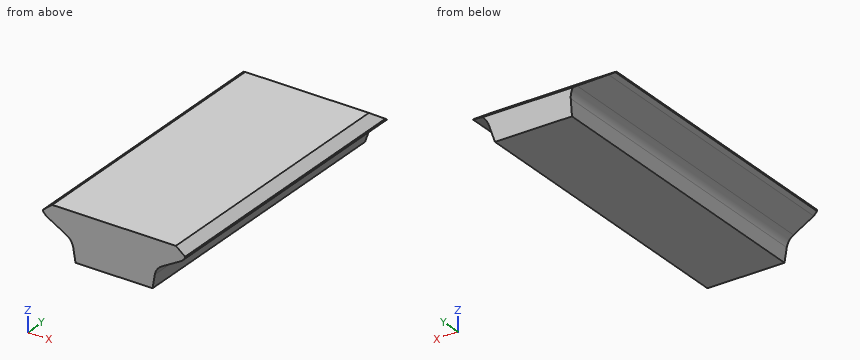
from build123d import *

# Parameters (mm, degrees)
F1_DEPTH    = 459.4
F2_SIZE2    = 31.5
F2_SIZE     = 11.8
F3_T1_DEPTH = 453.6970794399
F4_R        = 20


# Not quite as in the source:
# - a fillet or chamfer that OpenCascade refuses, or shapes differently, is made with other operations: its cross-section is extruded or revolved along the edge and cut away or added


with BuildPart() as f1:
    # F0 (on Front) → F1 (new body)
    with BuildSketch(Plane.XZ):
        Polygon((-61.18, 29.2), (-56.25, 0), (56.25, 0), (61.18, 29.2), (99, 50.6), (103.7, 55.8), (103.7, 57.8), (90.23, 68.48), (-90.23, 68.48), (-103.7, 57.8), (-103.7, 55.8), (-99, 50.6), align=None)
    extrude(amount=F1_DEPTH)

    # F2
    f2_edges = [f1.edges().sort_by_distance(p)[0] for p in [
        (0, 0, 0),
    ]]
    f2_side = f1.faces().sort_by_distance((0, -229.7, 0))[0]
    chamfer(f2_edges, length=F2_SIZE, length2=F2_SIZE2, reference=f2_side)

    # F3: chamfer of 52.9 x 37 on 1 edges, made by hand

    # F3_s2 → F3_t1 (cut)
    with BuildSketch(Plane.YZ.offset(-226.8485397199)):
        Polygon((0, 31.48), (-52.9, 68.48), (0, 68.48), align=None)
    extrude(amount=F3_T1_DEPTH, mode=Mode.SUBTRACT)

    # F4 (call 1 of 2: OpenCascade refuses the feature's edges together)
    f4_edges = [f1.edges().sort_by_distance(p)[0] for p in [
        (61.18, -230.130794, 29.2),
    ]]
    fillet(f4_edges, radius=F4_R)

    # F4#2 (call 2 of 2)
    f4_2_edges = [f1.edges().sort_by_distance(p)[0] for p in [
        (-61.18, -230.130794, 29.2),
    ]]
    fillet(f4_2_edges, radius=F4_R)


solid = f1.part
Source: CAD feature listing. Evaluate the final solid. Frame: model axes, mm. Round coordinates to 2 decimals unless told otherwise and drop trailing zeros. Loops run counter-clockwise (first coordinate to the right, second up) from the corner with the lowest first, then second, coordinate; pieces in that order, holes last. Notation, with made-up numbers: (49, 64) -> (67, 64) arc R13 ccw to (67, 85) -> close; hole circle Ø9 at (33.5, 25). An arc over 180 degrees is marked (long way). Answer as a JSON object with one key per item and string values. Group by question number.
Q1. Section query A-A (y = -374). Output: boundary loops of the cut face in (x, z), plus the area to 3 significant figures.
Q2. Ray query, line 1 (Y direction, x = 3.5, z = 36.5); line 2 (X direction, y = -176, z = 27.5); line 3 (Y direction, x = 57, z = 44.5). Return the intervals inside material, ascending. Write a range as from..to.
Q3. Section query B-B (x = 15). Output: boundary loops of the cut face in (y, z), plus the area to 3 significant figures.
Q4. Section query D-D (x = 83). Output: boundary loops of the cut face in (y, z).
Q5. Contact query for flat-ended pins moving along their axis: P1, Ø10, axis at y = -78.5, z = 34, coming from the +X side; P2, Ø3, axis at y = -361, z = 28.5, coming from the +X side; P3, Ø6, axis at y = -367.5, z = 10, coming from the -X side. Output: stop coordinate, or through.
Q6. Section query C-C (z = 8). Output: boundary loops of the cut face in (x, y).
Completed:
{
 "1": {"outline": "(-103.7, 55.8) -> (-99, 50.6) -> (-69.47, 33.89) arc R20 cw to (-59.59, 19.81) -> (-56.25, 0) -> (56.25, 0) -> (59.59, 19.81) arc R20 cw to (69.47, 33.89) -> (99, 50.6) -> (103.7, 55.8) -> (103.7, 57.8) -> (90.23, 68.48) -> (-90.23, 68.48) -> (-103.7, 57.8) -> close", "area": "10,400 mm²"},
 "2": {"line 1": "-459.4..-7.18", "line 2": "-62.62..62.62", "line 3": "-459.4..-18.62"},
 "3": {"outline": "(-459.4, 0) -> (-11.8, 0) -> (-0.01, 31.48) -> (-52.9, 68.48) -> (-459.4, 68.48) -> close", "area": "30,300 mm²"},
 "4": {"outline": "(-459.4, 41.55) -> (-14.39, 41.55) -> (-52.9, 68.48) -> (-459.4, 68.48) -> close"},
 "5": {"P1": "x = 78.5", "P2": "x = 64.58", "P3": "x = -58.44"},
 "6": {"outline": "(-57.6, -459.4) -> (57.6, -459.4) -> (57.6, -8.8) -> (-57.6, -8.8) -> close"}
}
